Check sheet for the modelled part. Datum: model origin and axes. Units: mm. A direction names the side the tool comes from. Round coordinates to 2 decimals unless told otherwise and drop trailing zeros. Write each loop counter-clockwise with the first axis right and the second up, starting at its lowest first coordinate (ties: lowest second). Pieces come first, ordered by that corner, then holes.
Item 1: Cross-section at A-A on x = 0. Enter the section's corners in (y, z), plus the area to 3 significant figures.
Item 2: Tool access check on faces 1 (the flat face through (0, -5, 280)), 2 (the flat face through (0, 15, 148)). Record the directions out of +Z, -Z, +X, -X, +Y, -Y that give a thin tool (end or side, any length) a straight path to the whole face; none if there is none.
Item 3: Go/stop test with a flat-tipped pin: pin 1 Ø16 at (x, z) = (0, 280) entering from -Y. Record where the tip stops, or that it passes through.
Item 4: Material ranges on line 1 (Z direction, x = 0, y = -7.75); line 2 (Z direction, x = -1, y = -9), recorded low to high.
Item 5: Cross-section at C-C on z = 280. Enter the section's corners in (x, y), plus the area to 3 significant figures.
Item 6: Release check for a two-part mould opening along Z. For faces 3 (the flat face through (15, 0, 148)), 4 (the flat face through (0, 0, 0)), 5 (the flat face through (0, 0, 300)), 6 (the cylindrical face through (-2.17, -10.07, 270.24)) record: +Z half, -Z half, draft (parallel to the pull), parting line (faces both ways), or undercut.
Item 7: Cross-section at B-B on y = -12.5. Enter the section's corners in (x, z), plus the area to 3 significant figures.
from build123d import *

# Parameters (mm, degrees)
SKETCH1_W           = 30
SKETCH1_H           = 30
BOSS_EXTRUDE1_DEPTH = 300
SKETCH2_R           = 10
CUT_EXTRUDE1_DEPTH  = 10


with BuildPart() as part:
    # Sketch1 → Boss-Extrude1 (new body)
    with BuildSketch(Plane.XY):
        Rectangle(SKETCH1_W, SKETCH1_H)
    extrude(amount=BOSS_EXTRUDE1_DEPTH)

    # Sketch2 → Cut-Extrude1 (cut)
    with BuildSketch(Plane.XZ.offset(15)):
        with Locations((0, 280)):
            Circle(SKETCH2_R)
    extrude(amount=-CUT_EXTRUDE1_DEPTH, mode=Mode.SUBTRACT)


solid = part.part
Response values:
1. outline: (-15, 0) - (15, 0) - (15, 300) - (-15, 300) - (-15, 290) - (-5, 290) - (-5, 270) - (-15, 270) - close
1. area: 8,800 mm2
2. face 1: -Y
2. face 2: +Z, -Z, +X, -X, +Y
3. pin 1: stops at y = -5
4. line 1: z = 0 to 270, 290 to 300
4. line 2: z = 0 to 270.05, 289.95 to 300
5. outline: (-15, -15) - (-10, -15) - (-10, -5) - (10, -5) - (10, -15) - (15, -15) - (15, 15) - (-15, 15) - close
5. area: 700 mm2
6. face 3: draft
6. face 4: -Z half
6. face 5: +Z half
6. face 6: undercut
7. outline: (-15, 0) - (15, 0) - (15, 300) - (-15, 300) - close; hole circle Ø20 at (0, 280)
7. area: 8,690 mm2
